The listing builds one solid part. Answer for the finished solid, in the listing's coordinates (mm). A direction names the side the tool comes from. Round coordinates to 2 decimals unless told otherwise and drop trailing zeros. Order: outer loops, then holes, each group sorted by start corner. A loop starts at its lowest first (then second) coordinate and runs counter-clockwise, first axis right, second up. Notation, with made-up numbers: (-16, 4.25) - (0, 4.25) arc R16 cw to (0, 12.25) - close; hole circle Ø3 at (36.5, 62.25). An arc over 180 degrees is marked (long way). One line per item, written item: value. Start each with the question number.
1. Flat-ended cylindrical pins translate along their axes: P1, Ø8.5, axis at y = -3.5, z = -29, coming from the -X side; P2, Ø2, axis at x = -3.5, y = 0, coming from the +Z side (3 decimals); P3, Ø12, axis at y = 2.5, z = -15.5, coming from the +X side; P4, Ø1, axis at x = 8.5, y = -1, coming from the -Z side. Find the tip coordinate at first contact, or state that the pin passes through.
2. Straight lines are drawn through the part: line 1 (X direction, y = -6.5, z = 14) (3 decimals); line 2 (Y direction, x = -6, z = 9.5) (1 decimal); line 3 (Z direction, x = -14, y = -3.5) (3 decimals). For each, find the intervals that lie inside material, in ascending order.
3. Section A-A, the plane y = 0 is taken. Give the vertices of the cut face in (x, z) (3 decimals), then the cut area to 3 significant figures.
4. Section C-C, the plane x = 17 is taken. Give the vertices of the cut face in (y, z) (1 decimal).
5. For a pull along X with two mould halves and no side action, classify faces 1 (the flat face through (0, -12.764, 16)), 2 (the flat face through (13.97, 7, -14)), 3 (the flat face through (13, 0, 28.575)), 4 (the flat face through (0, 12.764, 16)) as released by +X, released by -X, zero draft, split by the parting line, or undercut.
6. Section D-D, the plane z = -22 is taken. Give the vertices of the cut face in (x, y), then the cut area to 3 significant figures.
7. A tool of negligible diameter and unlimited length cuts with its end or side. For faces 5 (the flat face through (12.827, -3, 19)), 6 (the flat face through (-6, 0, 0)), 7 (the flat face through (19.05, 0, 3)), 8 (the cylindrical face through (15.982, 0.141, 19.072)), 9 (the cylindrical face through (16.55, 3.39, -34.57)), from which of +Z, -Z, +X, -X, +Y, -Y can it reach the whole face along a straight path? Write none if from no direction.
from build123d import *
from OCP.BRepFilletAPI import BRepFilletAPI_MakeChamfer

# Parameters (mm, degrees)
SKETCH1_W           = 31.75
SKETCH1_H           = 31.75
BOSS_EXTRUDE1_DEPTH = 28.575
SKETCH2_W           = 25.654
SKETCH2_H           = 25.527
CUT_EXTRUDE1_DEPTH  = 25.4
BOSS_EXTRUDE2_DEPTH = 3.175
BOSS_EXTRUDE3_DEPTH = 1.905
FILLET1_R           = 9.525
CUT_EXTRUDE2_REACH  = 56.068
SKETCH6_R           = 11.2776
SKETCH6_R_2         = 3.2004
CHAMFER1_SIZE       = 3.81
CHAMFER1_SIZE2      = 3.979101764


with BuildPart() as part:
    # Sketch1 → Boss-Extrude1 (new body)
    with BuildSketch(Plane.XY):
        Rectangle(SKETCH1_W, SKETCH1_H)
    extrude(amount=BOSS_EXTRUDE1_DEPTH)

    # Sketch2 → Cut-Extrude1 (cut)
    with BuildSketch(Plane.XY.offset(28.575)):
        Rectangle(SKETCH2_W, SKETCH2_H)
    extrude(amount=-CUT_EXTRUDE1_DEPTH, mode=Mode.SUBTRACT)

    # Sketch4 → Boss-Extrude2 (add)
    with BuildSketch(Plane(origin=(15.875, 0, 0), x_dir=(0, 0, -1), z_dir=(1, 0, 0))):
        Polygon((-28.575, -15.875), (0, -15.875), (38.1, -14.2875), (38.1, 14.2875), (0, 15.875), (-28.575, 15.875), align=None)
    extrude(amount=BOSS_EXTRUDE2_DEPTH)

    # Sketch5 → Boss-Extrude3 (add)
    with BuildSketch(Plane.ZY.offset(-15.875)):
        Polygon((-38.1, -14.2875), (0, -15.875), (0, 15.875), (-38.1, 14.2875), align=None)
    extrude(amount=BOSS_EXTRUDE3_DEPTH)

    # Fillet1
    # the kernel refuses this fillet: 9.525 mm, written as the material it adds along each edge
    with BuildSketch(Plane(origin=(13.97, -15.875, 0), x_dir=(-1, 0, 0), z_dir=(0, 1, 0))) as fillet1_piece_1_section:
        with BuildLine():
            CenterArc((FILLET1_R, -FILLET1_R), FILLET1_R, 90, 90)
            Line((0, -FILLET1_R), (0, 0))
            Line((0, 0), (FILLET1_R, 0))
        make_face()
    fillet1_piece_1 = extrude(amount=31.75, mode=Mode.PRIVATE)
    fillet1_piece_1 = split(fillet1_piece_1, bisect_by=Plane(origin=(11.807061563, -15.758253216, -2.801922808), z_dir=(0, 0.999133073092352, 0.04163054471218078)), keep=Keep.TOP, mode=Mode.PRIVATE)
    fillet1_piece_1 = split(fillet1_piece_1, bisect_by=Plane(origin=(11.807061563, 15.758253216, -2.801922808), z_dir=(0, -0.9991330730923519, 0.041630544712181895)), keep=Keep.TOP, mode=Mode.PRIVATE)
    add(fillet1_piece_1)

    # Sketch6 → Cut-Extrude2 (cut, up to next)
    with BuildSketch(Plane(origin=(19.05, 0, 0), x_dir=(0, 0, -1), z_dir=(1, 0, 0)), mode=Mode.PRIVATE) as cut_extrude2_sk1:
        with Locations((23.8125, 0)):
            Circle(SKETCH6_R)
    cut_extrude2_tool1 = extrude(cut_extrude2_sk1.sketch, amount=-CUT_EXTRUDE2_REACH, mode=Mode.PRIVATE) & part.part
    # Sketch6 → Cut-Extrude2 (cut, up to next)
    with BuildSketch(Plane(origin=(19.05, 0, 0), x_dir=(0, 0, -1), z_dir=(1, 0, 0)), mode=Mode.PRIVATE) as cut_extrude2_sk2:
        with Locations((-15.875, 0)):
            Circle(SKETCH6_R_2)
    cut_extrude2_tool2 = extrude(cut_extrude2_sk2.sketch, amount=-CUT_EXTRUDE2_REACH, mode=Mode.PRIVATE) & part.part
    add(cut_extrude2_tool1.solids().sort_by_distance((19.05, 0, -23.8125))[0], mode=Mode.SUBTRACT)
    add(cut_extrude2_tool2.solids().sort_by_distance((19.05, 0, 15.875))[0], mode=Mode.SUBTRACT)

    # Chamfer1: one chamfer whose edges measure the first distance from different faces: ONE call of the kernel's chamfer builder (chamfer() names one face for all edges)
    chamfer1_edges_1 = [part.edges().sort_by_distance(p)[0] for p in [
        (16.51, -14.2875, -38.1),
    ]]
    chamfer1_side_1 = [part.faces().sort_by_distance(p)[0] for p in [
        (16.083382106, -15.145696386, -17.503286726),
    ]]
    chamfer1_edges_2 = [part.edges().sort_by_distance(p)[0] for p in [
        (16.51, 14.2875, -38.1),
    ]]
    chamfer1_side_2 = [part.faces().sort_by_distance(p)[0] for p in [
        (16.51, 0, -38.1),
    ]]
    chamfer1 = BRepFilletAPI_MakeChamfer(part.part.solid().wrapped)
    for e in chamfer1_edges_1:
        chamfer1.Add(CHAMFER1_SIZE, CHAMFER1_SIZE2, e.wrapped, chamfer1_side_1[0].wrapped)  # the first distance lies on this face
    for e in chamfer1_edges_2:
        chamfer1.Add(CHAMFER1_SIZE, CHAMFER1_SIZE2, e.wrapped, chamfer1_side_2[0].wrapped)  # the first distance lies on this face
    add(Compound.cast(chamfer1.Shape()), mode=Mode.REPLACE)


solid = part.part
Answer list:
1. P1: passes through
1. P2: stops at z = 3.175
1. P3: stops at x = 19.05
1. P4: stops at z = -1.16
2. line 1: x = -15.875 to -12.827, 12.827 to 19.05
2. line 2: y = -15.9 to -12.8, 12.8 to 15.9
2. line 3: z = 0 to 28.575
3. outline: (-15.875, 0) - (4.445, 0) arc R9.525 cw to (13.97, -9.525) - (13.97, -12.535) - (19.05, -12.535) - (19.05, 12.675) - (12.827, 12.675) - (12.827, 3.175) - (-12.827, 3.175) - (-12.827, 28.575) - (-15.875, 28.575) - close; (12.827, 19.075) - (19.05, 19.075) - (19.05, 28.575) - (12.827, 28.575) - close; (13.97, -38.1) - (19.05, -38.1) - (19.05, -35.09) - (13.97, -35.09) - close
3. area: 405 mm²
4. outline: (-15.9, 0) - (-14.4, -34.3) - (-10.3, -38.1) - (10.5, -38.1) - (14.5, -34.1) - (15.9, 0) - (15.9, 28.6) - (-15.9, 28.6) - close; hole circle Ø22.6 at (0, -23.8); hole circle Ø6.4 at (0, 15.9)
5. face 1: undercut
5. face 2: released by -X
5. face 3: zero draft
5. face 4: undercut
6. outline: (13.97, -14.96) - (19.05, -14.96) - (19.05, -11.13) - (13.97, -11.13) - close; (13.97, 11.13) - (19.05, 11.13) - (19.05, 14.96) - (13.97, 14.96) - close
6. area: 38.9 mm²
7. face 5: +Z
7. face 6: -Z, -X, +Y, -Y
7. face 7: +Z, -Z, +X, +Y, -Y
7. face 8: +X
7. face 9: +X, -X
